Autodesk Inventor part; units mm, degrees
ref_plane "YZ Plane" through (0, 0, 0) normal (1, 0, 0) x (0, 1, 0)
ref_plane "XZ Plane" through (0, 0, 0) normal (0, 1, 0) x (-1, 0, 0)
ref_plane "XY Plane" through (0, 0, 0) normal (0, 0, 1) x (1, 0, 0)
sketch "スケッチ1" plane through (0, 0, 0) normal (0, 0, 1) x (1, 0, 0)
  circle A0 centre (0, 0) radius 4
  dimension "d13" = 8
extrude "押し出し1" add sketch "スケッチ1" along normal blind 60
sketch "スケッチ2" plane through (0, 0, 60) normal (0, 0, 1) x (1, 0, 0)
  point P0 (0, 0)
  point P1 (0, 0)
hole "穴1" at (0, 0, 60) direction (0, 0, -1) diameter 3.242 end through all
chamfer "面取り1" distance 0.2 angle 45 4 edges at (0, 1.621, 60) (0, 1.621, 0) (-4, 0, 60) (-4, 0, 0)
properties part number "ARF-4_1" material "鋼、炭素鋼"
Can you work these out from the model? Positions are in its coordinate system, mm. Round coordinates to 2 decimals unless told otherwise and drop trailing zeros. Loops run counter-clockwise (first coordinate to the right, second up) from the corner with the lowest first, then second, coordinate; pieces in that order, holes last. Notation, with made-up numbers: (36.5, 85.5) - (54.5, 85.5) arc R17 ccw to (54.5, 99.5) - close; hole circle Ø7 at (-28.5, -7.75). An arc over 180 degrees is marked (long way). Use CSV: the item, a comma, the result in double quotes. Start each with the question number.
1) For pin 1 Ø1.5 at (x, z) = (1.5, 9) entering from -Y; pin 2 Ø3 at (x, y) = (0, 0) entering from -Z, each with a flat end and sliding along its axis, tell me the tip position at first contact or that it passes through.
2) We'd pull the mould along Y, two halves only. Please class faces 1 (the flat face through (2, 1, 60)), 2 (the cylindrical face through (1.438, -0.748, 29.583)), 3 (the cylindrical face through (-0.867, 3.905, 29.583)): released by +Y, released by -Y, zero draft, split by the parting line, or undercut.
3) If we section it at C-C on z = 47.5: Write out the boundary of the cut face in (x, y), plus the area to 3 significant figures.
4) If we section it at A-A on y = 0: Write out the boundary of the cut face in (x, z).
5) Please list where these lines run through material, in increasing order: probe 1 along Y at (x, z) = (0, 29.5); probe 2 along X at (y, z) = (-0.5, 43.5). Write a range as [from, to].
Geometry results:
1,pin 1,"stops at y = -3.93"
1,pin 2,"passes through"
2,face 1,"zero draft"
2,face 2,"undercut"
2,face 3,"split by the parting line"
3,outline,"circle Ø8 at (0, 0); hole circle Ø3.24 at (0, 0)"
3,area,"42.0 mm2"
4,outline,"(-4, 0.2) - (-3.8, 0) - (-1.82, 0) - (-1.62, 0.2) - (-1.62, 59.8) - (-1.82, 60) - (-3.8, 60) - (-4, 59.8) - close; (1.62, 0.2) - (1.82, 0) - (3.8, 0) - (4, 0.2) - (4, 59.8) - (3.8, 60) - (1.82, 60) - (1.62, 59.8) - close"
5,probe 1,"y = [-4, -1.62], [1.62, 4]"
5,probe 2,"x = [-3.97, -1.54], [1.54, 3.97]"
